The listing builds one solid part. Answer for the finished solid, in the listing's coordinates (mm). A direction names the side the tool comes from. Round coordinates to 2 decimals unless told otherwise and drop trailing zeros. Write each loop counter-clockwise with the first axis right and the second up, starting at its lowest first coordinate (ties: lowest second). Pieces come first, ordered by that corner, then holes.
(1) The mould has two halves that part along Z. Classify faces 1 (the face through (-0.75, 9.4, 4.7)), 2 (the face through (0.75, -9.5, 3.2)), 3 (the face through (7.3, 0, 0)), 4 (the face through (0, -4, 7.5)): +Z half, -Z half, draft (parallel to the pull), parting line (faces both ways), or undercut.
(2) A cutting plane is placed at A-A, the plane z = 1.75. Give the vertices of the cut face in (x, y), and give its area (3 significant figures).
(3) A cutting plane is placed at D-D, the plane x = 6.5. Give the vertices of the cut face in (y, z), and give its area (3 significant figures).
(4) Find the intervals of material crossed by probe 1 along X at (y, z) = (2.5, 2.75); probe 2 along Y at (x, z) = (0, 6.4); probe 3 along X at (y, z) = (-1.5, 2.25), in increasing order.
(5) For faces 5 (the face through (-0.75, -9.4, 3.2)), 6 (the face through (-9.5, -0.75, 3)), 7 (the face through (-7.14, -7, 2.96)), determine the directions among +Z, -Z, +X, -X, +Y, -Y from which every point of the face is accessible in a straight line to the end or side of a thin tool.
(6) A cutting plane is placed at C-C, the plane x = -1.5. Give the vertices of the cut face in (y, z).
(7) Each of these flat-tipped pins is pushed along its axis until it touches: pin 1 Ø0.5 at (y, z) = (-9.5, 4) entering from -X; pin 2 Ø2 at (y, z) = (9, 5.5) entering from +X; pin 3 Ø1.5 at (x, z) = (-6, 5.5) entering from +Y. Where does it stop, or does it pass through?
(8) A cutting plane is placed at B-B, the plane y = 0. Give the vertices of the cut face in (x, z).
from build123d import *

# Parameters (mm, degrees)
SKETCH1_R           = 10
SKETCH1_R_2         = 3.25
BOSS_EXTRUDE1_DEPTH = 7.5
SKETCH2_R           = 9
CUT_EXTRUDE1_DEPTH  = 6
CUT_EXTRUDE2_DEPTH  = 6
CIRPATTERN1_COUNT   = 3
CIRPATTERN1_ANGLE   = 180
BOSS_EXTRUDE2_DEPTH = 6
CUT_EXTRUDE3_DEPTH  = 0.5
BOSS_EXTRUDE3_DEPTH = 3.5
BOSS_EXTRUDE4_DEPTH = 3
SKETCH8_R           = 17.5
SKETCH8_R_2         = 10
BOSS_EXTRUDE5_DEPTH = 1.5


with BuildPart() as part:
    # Sketch1 → Boss-Extrude1 (new body)
    with BuildSketch(Plane.XY):
        Circle(SKETCH1_R)
        Circle(SKETCH1_R_2, mode=Mode.SUBTRACT)
    extrude(amount=BOSS_EXTRUDE1_DEPTH)

    # Sketch2 → Cut-Extrude1 (cut)
    with BuildSketch(Plane.XY):
        Circle(SKETCH2_R)
    extrude(amount=CUT_EXTRUDE1_DEPTH, mode=Mode.SUBTRACT)

    # Sketch3 → Cut-Extrude2 (cut)
    with BuildSketch(Plane(origin=(0, 0, 0), x_dir=(-1, 0, 0), z_dir=(0, 0, -1))):
        with BuildLine():
            Line((0.75, -9.971835338), (0.75, -8.968695557))
            ThreePointArc((0.75, -8.968695557), (0, -9), (-0.75, -8.968695557))
            Line((-0.75, -8.968695557), (-0.75, -9.971835338))
            ThreePointArc((-0.75, -9.971835338), (0, -10), (0.75, -9.971835338))
        make_face()
    cut_extrude2 = extrude(amount=-CUT_EXTRUDE2_DEPTH, mode=Mode.SUBTRACT)

    # CirPattern1: Cut-Extrude2 ×3 about axis
    cirpattern1_axis = Axis((0, 0, 0), (0, 0, -1))
    for i in range(1, CIRPATTERN1_COUNT):
        add(cut_extrude2.rotate(cirpattern1_axis, i * CIRPATTERN1_ANGLE / (CIRPATTERN1_COUNT - 1)), mode=Mode.SUBTRACT)

    # Sketch4 → Boss-Extrude2 (add)
    with BuildSketch(Plane(origin=(0, 0, 6), x_dir=(-1, 0, 0), z_dir=(0, 0, -1))):
        with BuildLine():
            Line((-2.736161147, 7.517540966), (-2.394141003, 6.577848346))
            ThreePointArc((-2.394141003, 6.577848346), (-7, 0), (-2.394141003, -6.577848346))
            Line((-2.394141003, -6.577848346), (-2.736161147, -7.517540966))
            ThreePointArc((-2.736161147, -7.517540966), (-8, 0), (-2.736161147, 7.517540966))
        make_face()
    extrude(amount=BOSS_EXTRUDE2_DEPTH)

    # Sketch5 → Cut-Extrude3 (cut)
    with BuildSketch(Plane(origin=(0, 0, 6), x_dir=(-1, 0, 0), z_dir=(0, 0, -1))):
        with BuildLine():
            Line((-0.75, -8.968695557), (-0.75, -9.971835338))
            ThreePointArc((-0.75, -9.971835338), (0, -10), (0.75, -9.971835338))
            Line((0.75, -9.971835338), (0.75, -7.964766161))
            ThreePointArc((0.75, -7.964766161), (-8, 0), (0.75, 7.964766161))
            Line((0.75, 7.964766161), (0.75, 9.971835338))
            ThreePointArc((0.75, 9.971835338), (0, 10), (-0.75, 9.971835338))
            Line((-0.75, 9.971835338), (-0.75, 8.968695557))
            ThreePointArc((-0.75, 8.968695557), (-9, 0), (-0.75, -8.968695557))
        make_face()
    extrude(amount=-CUT_EXTRUDE3_DEPTH, mode=Mode.SUBTRACT)

    # Sketch6 → Boss-Extrude3 (add)
    with BuildSketch(Plane(origin=(0, 0, 6.5), x_dir=(-1, 0, 0), z_dir=(0, 0, -1))):
        with BuildLine():
            Line((-0.75, 8.968695557), (-0.75, 9.971835338))
            ThreePointArc((-0.75, 9.971835338), (-0.500156715, 9.987484331), (-0.25, 9.996874512))
            Line((-0.25, 9.996874512), (-0.25, 8.996527108))
            ThreePointArc((-0.25, 8.996527108), (-0.500193611, 8.986089603), (-0.75, 8.968695557))
        make_face()
    extrude(amount=BOSS_EXTRUDE3_DEPTH)

    # Sketch7 → Boss-Extrude4 (add)
    with BuildSketch(Plane(origin=(0, 0, 3), x_dir=(-1, 0, 0), z_dir=(0, 0, -1))):
        with BuildLine():
            ThreePointArc((0.25, 8.996527108), (0.500193611, 8.986089603), (0.75, 8.968695557))
            Line((0.75, 8.968695557), (0.75, 9.971835338))
            ThreePointArc((0.75, 9.971835338), (0.500156715, 9.987484331), (0.25, 9.996874512))
            Line((0.25, 9.996874512), (0.25, 8.996527108))
        make_face()
    extrude(amount=BOSS_EXTRUDE4_DEPTH)

    # Sketch8 → Boss-Extrude5 (add)
    with BuildSketch(Plane.XY.offset(7.5)):
        Circle(SKETCH8_R)
        Circle(SKETCH8_R_2, mode=Mode.SUBTRACT)
    extrude(amount=-BOSS_EXTRUDE5_DEPTH)


solid = part.part
Solutions:
1. face 1: undercut
1. face 2: draft
1. face 3: -Z half
1. face 4: +Z half
2. outline: (-9.97, -0.75) arc R10 ccw to (-0.75, -9.97) - (-0.75, -8.97) arc R9 cw to (-8.97, -0.75) - close; (-9.97, 0.75) - (-8.97, 0.75) arc R9 cw to (-0.25, 9) - (-0.25, 10) arc R10 ccw to (-0.75, 9.97) arc R10 ccw to start; (0.75, -9.97) arc R10 ccw to (0.75, 9.97) - (0.75, 8.97) arc R9 cw to (0.75, -8.97) - close; (2.39, -6.58) - (2.74, -7.52) arc R8 ccw to (2.74, 7.52) - (2.39, 6.58) arc R7 cw to start
2. area: 74.0 mm2
3. outline: (-16.25, 6) - (-7.6, 6) - (-7.6, 0) - (-6.22, 0) - (-6.22, 6.5) - (-4.66, 6.5) - (-4.66, 0) - (-2.6, 0) - (-2.6, 6) - (2.6, 6) - (2.6, 0) - (4.66, 0) - (4.66, 6.5) - (6.22, 6.5) - (6.22, 0) - (7.6, 0) - (7.6, 6) - (16.25, 6) - (16.25, 7.5) - (-16.25, 7.5) - close
3. area: 88.5 mm2
4. probe 1: x = -9.68 to -8.65, 6.54 to 7.6, 8.65 to 9.68
4. probe 2: y = -17.5 to -10, -8 to -3.25, 3.25 to 8, 10 to 17.5
4. probe 3: x = -9.89 to -8.87, 6.84 to 7.86, 8.87 to 9.89
5. face 5: -Z
5. face 6: -Z, -X
5. face 7: -Z, -X, -Y
6. outline: (-17.44, 6) - (-9.89, 6) - (-9.89, 0) - (-8.87, 0) - (-8.87, 6) - (-2.88, 6) - (-2.88, 7.5) - (-17.44, 7.5) - close; (2.88, 6) - (8.87, 6) - (8.87, 0) - (9.89, 0) - (9.89, 6) - (17.44, 6) - (17.44, 7.5) - (2.88, 7.5) - close
7. pin 1: stops at x = -3.8
7. pin 2: stops at x = 15.49
7. pin 3: stops at y = 16.63
8. outline: (-17.5, 6) - (-3.25, 6) - (-3.25, 7.5) - (-17.5, 7.5) - close; (3.25, 6) - (7, 6) - (7, 0) - (8, 0) - (8, 6.5) - (9, 6.5) - (9, 0) - (10, 0) - (10, 6) - (17.5, 6) - (17.5, 7.5) - (3.25, 7.5) - close
